Input: dimensioned drawing with shaded views. Units: mm. Origin: part minimum x, y, z. A direction names the side the tool comes from. Give positions to 0.01 mm unless a question says otherwise; leave off trailing zeros. Loops run counter-clockwise (first coordinate to the right, second up) from the corner with the lowest first, then second, coordinate; pieces in that order, holes last. Notation, with made-up numbers: (-37, 65.5) -> (16, 65.5) arc R17 ccw to (16, 71.5) -> close; hole circle Ø11 at (15.5, 8.25). An arc over 180 degrees is marked (long way). Answer in a Markdown table with one row per item. Add a question column.
1) Section query B-B (z = 32). Return the cut outline in (x, y), plus the area to 3 significant figures.
2) Section query A-A (x = 20). Return the cut outline in (y, z).
3) Access query for the marked faces 1 and 2. Directions: +Z, -Z, +X, -X, +Y, -Y. A direction counts if a zero-diameter tool reaches every point of the face in a straight line with its end or side. Return the directions, or none.
4) First-contact query: P1, Ø6, axis at x = 13, z = 29.5, coming from the +Y side; P2, Ø4, axis at x = 17.5, y = 35.5, coming from the -Z side; P3, Ø4, axis at x = 24.5, y = 18, coming from the +Z side. Flat tips, straight axial feed; report the tip coordinate or a pass-through.
5) Section query D-D (z = 13). Return the cut outline in (x, y) (1 decimal).
6) Line query: line 1 (Y direction, x = 20, z = 17.25); line 2 (Y direction, x = 34, z = 12); line 3 (Z direction, x = 20.5, y = 39). Output: solid intervals per line, ascending. Write a range as from..to.
7) Section query C-C (y = 9.5). Return the cut outline in (x, z).
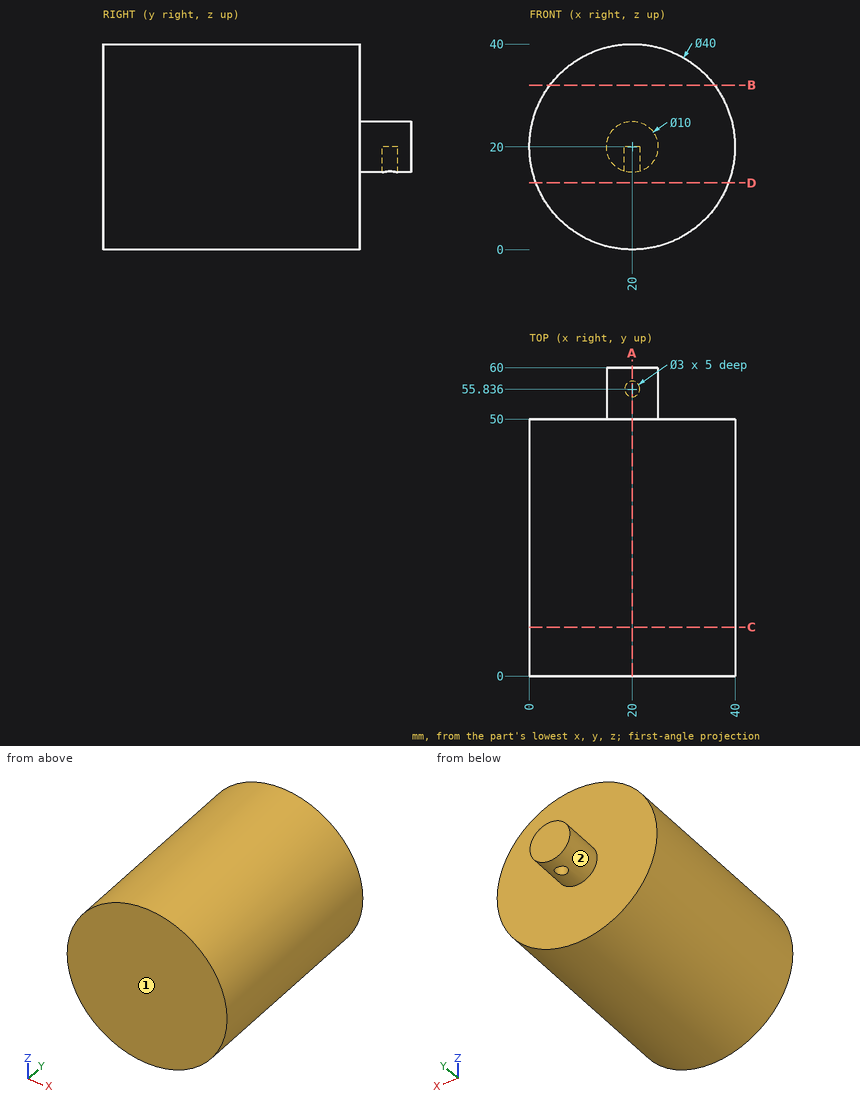
Evaluation:
| question | item | result |
|---|---|---|
| 1 | outline | (4, 0) -> (36, 0) -> (36, 50) -> (4, 50) -> close |
| 1 | area | 1,600 mm² |
| 2 | outline | (0, 0) -> (50, 0) -> (50, 15) -> (54.34, 15) -> (54.34, 20) -> (57.34, 20) -> (57.34, 15) -> (60, 15) -> (60, 25) -> (50, 25) -> (50, 40) -> (0, 40) -> close |
| 3 | face 1 | +Z, -Z, +X, -X, -Y |
| 3 | face 2 | +Y |
| 4 | P1 | y = 50 |
| 4 | P2 | z = 0.01 |
| 4 | P3 | z = 39.84 |
| 5 | outline | (1.3, 0) -> (38.7, 0) -> (38.7, 50) -> (1.3, 50) -> close |
| 6 | line 1 | 0..54.34, 57.34..60 |
| 6 | line 2 | 0..50 |
| 6 | line 3 | 0.01..39.99 |
| 7 | outline | circle Ø40 at (20, 20) |
